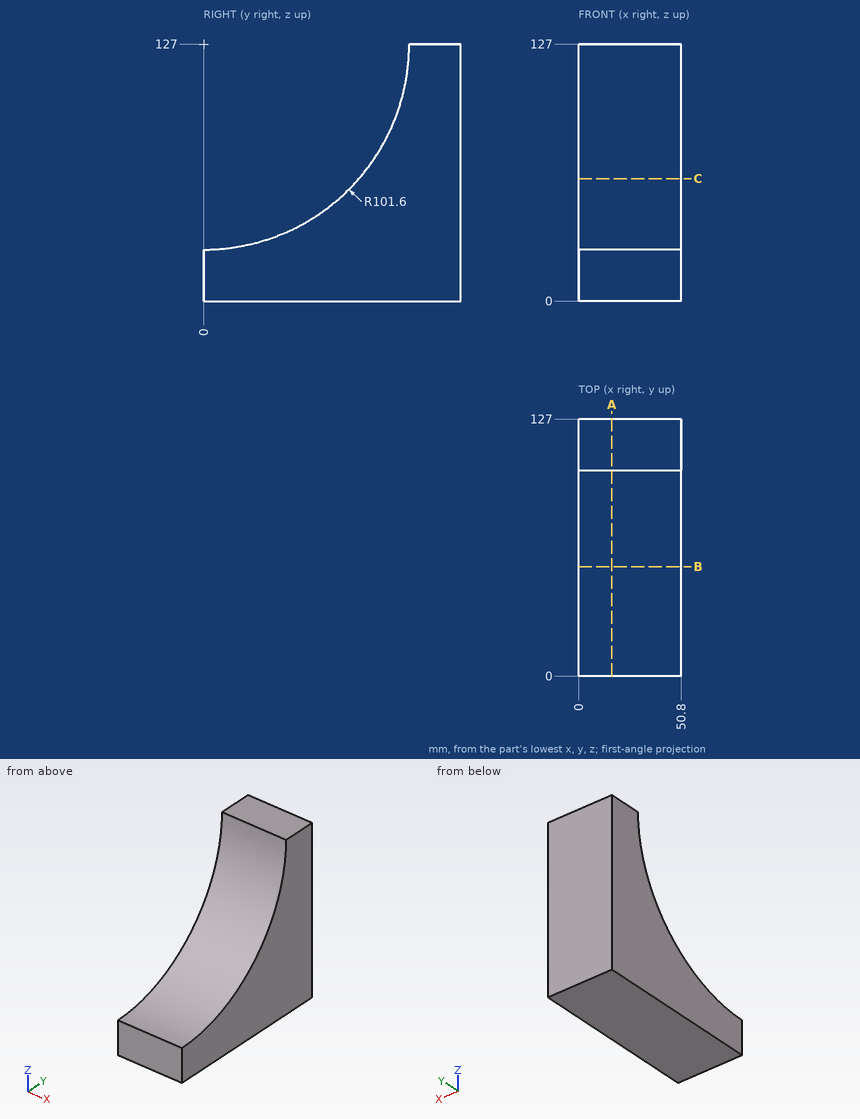
Could you check a few things on this drawing? It's one solid part, dimensions in mm from its lowest x, y, z. Give positions to 0.01 mm unless a question says otherwise; leave off trailing zeros. Write each loop counter-clockwise with the first axis right and the second up, starting at its lowest first coordinate (ties: lowest second). Pieces come first, ordered by that corner, then holes.
(1) If I drill on L1, parallel to Z at x = 34, y = 64; L2, parallel to Z at x = 21.5, y = 7.5; L3, parallel to Y at x = 39.5, z = 55, over which ranges is the centre line in solid material (lowest first)?
Output values:
L1: z = 0 to 48.09
L2: z = 0 to 25.68
L3: y = 71.68 to 127
(2) Will these pins go through, and if not, where does the flat tip stop? pin 1 (5 mm diameter, centred on x = 45.5, y = 73, fed in from +Z); pin 2 (8 mm diameter, centred on x = 9, z = 41.5, fed in from -Y); pin 3 (8 mm diameter, centred on x = 24.5, y = 70.5, fed in from +Z).
Output values:
pin 1: stops at z = 59.01
pin 2: stops at y = 48.09
pin 3: stops at z = 57.92
(3) Imagine slicing it at C-C, the plane z = 60.5. Write out the boundary of the cut face in (x, y).
Output values:
outline: (0, 76.81) - (50.8, 76.81) - (50.8, 127) - (0, 127) - close
(4) Imagine slicing it at A-A, the plane x = 16.5. Write out the boundary of the cut face in (y, z), and give its area (3 significant figures).
Output values:
outline: (0, 0) - (127, 0) - (127, 127) - (101.6, 127) arc R101.6 cw to (0, 25.4) - close
area: 8,020 mm2
(5) Imagine slicing it at B-B, the plane y = 54. Write out the boundary of the cut face in (x, z).
Output values:
outline: (0, 0) - (50.8, 0) - (50.8, 40.94) - (0, 40.94) - close
